For this review, take the finished solid that the model builds, in its own axes (mm). Round coordinates to 2 decimals unless told otherwise and drop trailing zeros. Write each loop counter-clockwise with the first axis right and the second up, starting at its lowest first coordinate (ties: lowest second). Pieces come first, ordered by that corner, then holes. Notation, with made-up numbers: M 70,65 L 97,65 A27 ccw 97,101 Z; hole C 41,66 d9. An arc over 180 degrees is marked long. Answer in a Markdown table with one row per item.
```python
from build123d import *

# Parameters (mm, degrees)
SKETCH1_R           = 1.5
SKETCH1_R_2         = 5
SKETCH1_R_3         = 10
BOSS_EXTRUDE2_DEPTH = 3


with BuildPart() as part:
    # Sketch1 → Boss-Extrude2 (new body)
    with BuildSketch(Plane(origin=(0, 0, 0), x_dir=(1, 0, 0), z_dir=(0, 1, 0))):
        Polygon((-71.5, 92.5), (-180, 92.5), (-180, -92.5), (-71.5, -92.5), (-71.5, -105), (-50, -105), (-50, -135), (50, -135), (50, -105), (71.5, -105), (71.5, -92.5), (180, -92.5), (180, 92.5), (71.5, 92.5), (71.5, 105), (50, 105), (50, 135), (-50, 135), (-50, 105), (-71.5, 105), align=None)
        with Locations((133, -70)):
            Circle(SKETCH1_R, mode=Mode.SUBTRACT)
        with Locations((120, -70)):
            Circle(SKETCH1_R, mode=Mode.SUBTRACT)
        with Locations((133, -82.5)):
            Circle(SKETCH1_R, mode=Mode.SUBTRACT)
        with Locations((120, -82.5)):
            Circle(SKETCH1_R, mode=Mode.SUBTRACT)
        with Locations((-120, -82.5)):
            Circle(SKETCH1_R, mode=Mode.SUBTRACT)
        with Locations((-133, -82.5)):
            Circle(SKETCH1_R, mode=Mode.SUBTRACT)
        with Locations((-120, -70)):
            Circle(SKETCH1_R, mode=Mode.SUBTRACT)
        with Locations((-133, -70)):
            Circle(SKETCH1_R, mode=Mode.SUBTRACT)
        with Locations((-133, 70)):
            Circle(SKETCH1_R, mode=Mode.SUBTRACT)
        with Locations((-120, 70)):
            Circle(SKETCH1_R, mode=Mode.SUBTRACT)
        with Locations((-133, 82.5)):
            Circle(SKETCH1_R, mode=Mode.SUBTRACT)
        with Locations((-120, 82.5)):
            Circle(SKETCH1_R, mode=Mode.SUBTRACT)
        with Locations((133, 82.5)):
            Circle(SKETCH1_R, mode=Mode.SUBTRACT)
        with Locations((120, 82.5)):
            Circle(SKETCH1_R, mode=Mode.SUBTRACT)
        with Locations((120, 70)):
            Circle(SKETCH1_R, mode=Mode.SUBTRACT)
        with Locations((133, 70)):
            Circle(SKETCH1_R, mode=Mode.SUBTRACT)
        with Locations((105.5, 22.5)):
            Circle(SKETCH1_R_2, mode=Mode.SUBTRACT)
        with Locations((105.5, -22.5)):
            Circle(SKETCH1_R_2, mode=Mode.SUBTRACT)
        with Locations((-105.5, -22.5)):
            Circle(SKETCH1_R_2, mode=Mode.SUBTRACT)
        with Locations((-105.5, 22.5)):
            Circle(SKETCH1_R_2, mode=Mode.SUBTRACT)
        with Locations((18.5, -55)):
            Circle(SKETCH1_R, mode=Mode.SUBTRACT)
        with Locations((-18.5, -55)):
            Circle(SKETCH1_R, mode=Mode.SUBTRACT)
        with Locations((18.5, -92)):
            Circle(SKETCH1_R, mode=Mode.SUBTRACT)
        with Locations((-18.5, -92)):
            Circle(SKETCH1_R, mode=Mode.SUBTRACT)
        with Locations((18.5, 92)):
            Circle(SKETCH1_R, mode=Mode.SUBTRACT)
        with Locations((-18.5, 92)):
            Circle(SKETCH1_R, mode=Mode.SUBTRACT)
        with Locations((-18.5, 55)):
            Circle(SKETCH1_R, mode=Mode.SUBTRACT)
        with Locations((18.5, 55)):
            Circle(SKETCH1_R, mode=Mode.SUBTRACT)
        with Locations((-40, -125)):
            Circle(SKETCH1_R_2, mode=Mode.SUBTRACT)
        with Locations((40, -125)):
            Circle(SKETCH1_R_2, mode=Mode.SUBTRACT)
        with Locations((40, 125)):
            Circle(SKETCH1_R_2, mode=Mode.SUBTRACT)
        with Locations((-40, 125)):
            Circle(SKETCH1_R_2, mode=Mode.SUBTRACT)
        with Locations((0, 115)):
            Circle(SKETCH1_R_3, mode=Mode.SUBTRACT)
        with Locations((0, -115)):
            Circle(SKETCH1_R_3, mode=Mode.SUBTRACT)
    extrude(amount=BOSS_EXTRUDE2_DEPTH)


solid = part.part
```
Q1. Take a section at A-A (x = 0). State the section outline as (y, z) points, then the cut area to 3 significant figures.
Found:
| item | result |
|---|---|
| outline | M 0,-135 L 3,-135 L 3,-125 L 0,-125 Z; M 0,-105 L 3,-105 L 3,105 L 0,105 Z; M 0,125 L 3,125 L 3,135 L 0,135 Z |
| area | 690 mm² |
Q2. Take a section at D-D (z = -101). State the section outline as (x, y) points, then the cut area to 3 significant figures.
Found:
| item | result |
|---|---|
| outline | M -71.5,0 L 71.5,0 L 71.5,3 L -71.5,3 Z |
| area | 429 mm² |
Q3. For probe 1 along X at (y, z) = (2.15, -82.5); probe 2 along Z at (x, y) = (18.5, 1.35); probe 3 along Z at (x, y) = (-133, 1.9), list the stretches that pass through material, from the lowest coordinate up.
Found:
| item | result |
|---|---|
| probe 1 | -180 to -134.5, -131.5 to -121.5, -118.5 to 118.5, 121.5 to 131.5, 134.5 to 180 |
| probe 2 | -135 to -93.5, -90.5 to -56.5, -53.5 to 53.5, 56.5 to 90.5, 93.5 to 135 |
| probe 3 | -92.5 to -84, -81 to -71.5, -68.5 to 68.5, 71.5 to 81, 84 to 92.5 |
Q4. Take a section at B-B (z = 22.5). State the section outline as (x, y) points.
Found:
| item | result |
|---|---|
| outline | M -180,0 L -110.5,0 L -110.5,3 L -180,3 Z; M -100.5,0 L 100.5,0 L 100.5,3 L -100.5,3 Z; M 110.5,0 L 180,0 L 180,3 L 110.5,3 Z |
Q5. Mouldability with a two-part tool opening along Z and no side actions: class faces 1 (the face through (-3, 3, -2)), 2 (the face through (-1.302, 1.479, 105.085)), 3 (the face through (110.119, 1.479, 24.415)) as +Z half, -Z half, draft (parallel to the pull), parting line (faces both ways), or undercut.
Found:
| item | result |
|---|---|
| face 1 | draft |
| face 2 | undercut |
| face 3 | undercut |
Q6. Insertion check: P1, Ø0.9, axis at x = -55.5, y = 1, coming from the +Z side; P2, Ø1.5, axis at y = 1.5, z = 118.5, coming from the -X side. Each pin has a flat end and moves straight along its axis. Give the tip position at first contact, or say it passes through.
Found:
| item | result |
|---|---|
| P1 | z = 105 |
| P2 | x = -50 |
Q7. Take a section at C-C (y = 1.9). State how many separate pieces and enclosed holes the cut face has, then the cut area to 3 significant figures.
Found:
| item | result |
|---|---|
| separate pieces | 1 |
| enclosed holes | 34 |
| area | 74,700 mm² |
